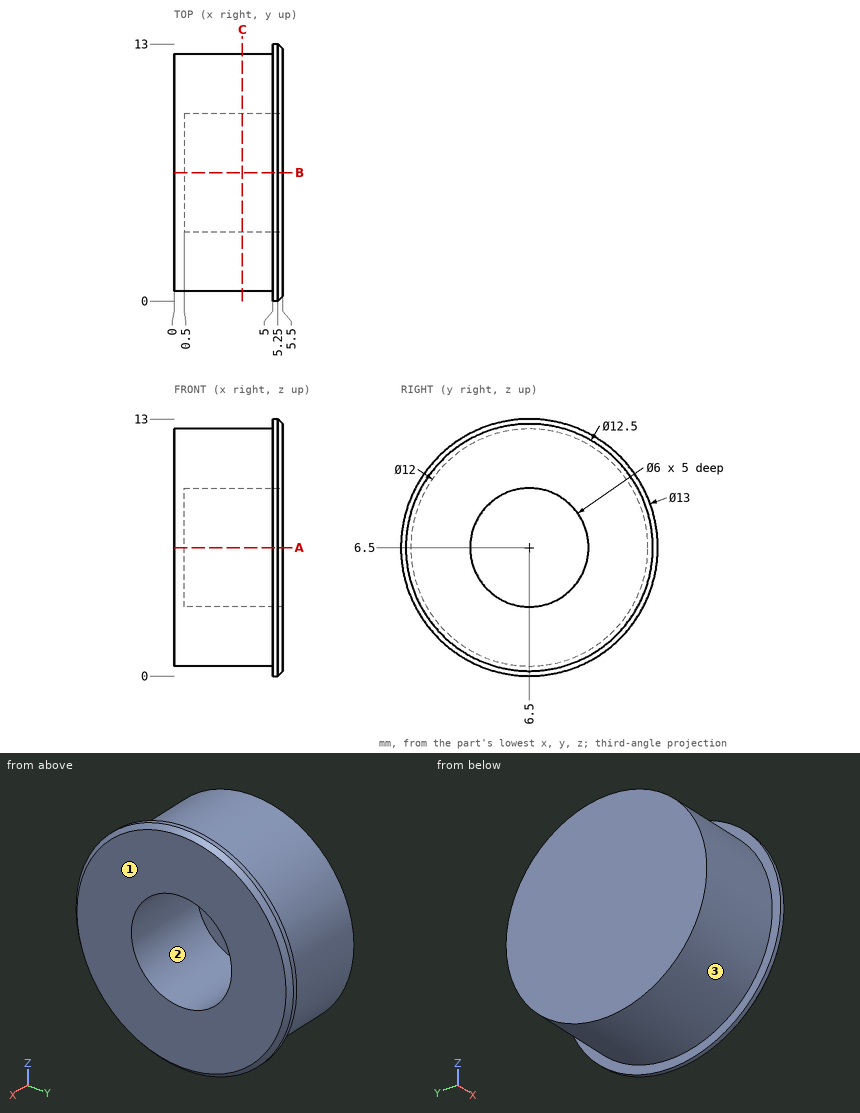
Here's the drawing with two shaded views (mm, measured from the low corner). I have some questions. Give positions to 0.01 mm unless a question says otherwise; leave off trailing zeros. Write each loop counter-clockwise with the first axis right and the second up, starting at its lowest first coordinate (ties: lowest second). Pieces come first, ordered by that corner, then holes. Notation, with made-up numbers: (4, 18) -> (32, 18) arc R17 ccw to (32, 45) -> close; hole circle Ø6 at (-22.5, -34). An arc over 180 degrees is marked (long way). Use one line per item in the form item = value. Start each with the question number.
1. Thinking about a two-plate mould opening in Y: for the marked faces 1, 2 and 3, which applies, +Y half, -Y half, draft (parallel to the pull), parting line (faces both ways), or undercut?
2. Imagine slicing it at C-C on x = 3.45. List the corners of the cut face in (y, z) for me.
3. Will these pins go through, and if not, where does the flat tip stop? pin 1 Ø1.5 at (x, y) = (1.5, 4.5) entering from -Z; pin 2 Ø6.5 at (y, z) = (9, 9) entering from -X.
4. Imagine slicing it at A-A on z = 6.5. List the corners of the cut face in (x, y) for me.
5. If I drill on L1, parallel to Z at x = 4.7, y = 9; L2, parallel to Z at x = 1.4, y = 6.75; L3, parallel to Y at x = 1.1, z = 5, over which ranges is the centre line in solid material (lowest first)?
Entries:
q1.face_1 = draft
q1.face_2 = undercut
q1.face_3 = parting line
q2.outline = circle Ø12 at (6.5, 6.5); hole circle Ø6 at (6.5, 6.5)
q3.pin_1 = 0.63
q3.pin_2 = 0
q4.outline = (0, 0.5) -> (5, 0.5) -> (5, 0) -> (5.25, 0) -> (5.5, 0.25) -> (5.5, 3.5) -> (0.5, 3.5) -> (0.5, 9.5) -> (5.5, 9.5) -> (5.5, 12.75) -> (5.25, 13) -> (5, 13) -> (5, 12.5) -> (0, 12.5) -> close
q5.L1 = 1.05 to 4.84, 8.16 to 11.95
q5.L2 = 0.51 to 3.51, 9.49 to 12.49
q5.L3 = 0.69 to 3.9, 9.1 to 12.31
